Here's how the part is built. I have some questions about the finished solid (model axes, mm). A direction names the side the tool comes from. Coordinates: 2 decimals unless noted, no trailing zeros. Order: outer loops, then holes, each group sorted by start corner. A loop starts at its lowest first (then second) coordinate and runs counter-clockwise, first axis right, second up. Notation, with made-up numbers: (-37.5, 69) - (-8.5, 69) arc R26 cw to (-8.5, 88) - close; hole circle Ø1 at (69.25, 15.5). An arc over 180 degrees is marked (long way). Answer as CSV lines item,"result". Start each with the question number.
Q1. For faces 1 (the face through (1, 46, 35)), 2 (the face through (-31.27, 39.03, 36.59)), which set-ups out of +Z, -Z, +X, -X, +Y, -Y let a thin tool reach every point of the face, with its end or its side?
Q2. For pin 1 Ø3.5 at (x, y) = (-45.75, 40) entering from +Z; pin 2 Ø10 at (x, y) = (-15, -26.5) entering from -Z, each with a flat end and sliding along its axis, tell me the tip position at first contact or that it passes through.
Q3. Suppose I cut it at B-B (x = 45.75). Please give me the cut outline in (y, z), then the cut area to 3 significant figures.
Q4. Suppose I cut it at C-C (z = 34.4). Please give me the cut outline in (x, y).
Q5. Suppose I cut it at D-D (y = 40). Please give me the cut outline in (x, z), then the cut area to 3 significant figures.
Q6. I need wall thicknesses on line 1 (X direction, y = -42, z = 36.5); line 2 (Y direction, x = -30, z = 36.6); line 3 (Y direction, x = 33, z = 33.95). Which ranges of each line are inside material? Lowest first, please.
Q7. Suppose I cut it at A-A (y = -42). Please give me the cut outline in (x, z).
Q8. Thinking about a two-plate mould opening in Y: for faces 3 (the face through (-1, -47, 35)), 4 (the face through (1, 47, 35)), 5 (the face through (-50.75, 1, 35)), 6 (the face through (49.75, -1, 35)), which applies, released by +Y, released by -Y, zero draft, split by the parting line, or undercut?
from build123d import *

# Parameters (mm, degrees)
PAD024_DEPTH    = 1
PAD025_DEPTH    = 3
SKETCH042_R     = 1.6
POCKET018_DEPTH = 5


with BuildPart() as part:
    # Sketch040 → Pad024 (new body)
    with BuildSketch(Plane.XY):
        with BuildLine():
            Line((-50.75, 46), (-50.75, -46))
            ThreePointArc((-50.75, -46), (-50.457107, -46.707107), (-49.75, -47))
            Line((-49.75, -47), (49.75, -47))
            ThreePointArc((49.75, -47), (50.457107, -46.707107), (50.75, -46))
            Line((50.75, -46), (50.75, 46))
            ThreePointArc((50.75, 46), (50.457107, 46.707107), (49.75, 47))
            Line((49.75, 47), (-49.75, 47))
            ThreePointArc((-49.75, 47), (-50.457107, 46.707107), (-50.75, 46))
        make_face()
    extrude(amount=PAD024_DEPTH)

    # Sketch041 → Pad025 (join)
    with BuildSketch(Plane.XY):
        with BuildLine():
            Line((-50.75, 46), (-50.75, -46))
            ThreePointArc((-50.75, -46), (-50.457107, -46.707107), (-49.75, -47))
            Line((-49.75, -47), (49.75, -47))
            ThreePointArc((49.75, -47), (50.457107, -46.707107), (50.75, -46))
            Line((50.75, -46), (50.75, 46))
            ThreePointArc((50.75, 46), (50.457107, 46.707107), (49.75, 47))
            Line((49.75, 47), (-49.75, 47))
            ThreePointArc((-49.75, 47), (-50.457107, 46.707107), (-50.75, 46))
        make_face()
        with BuildLine():
            Line((-49.75, 45), (-49.75, -45))
            ThreePointArc((-49.75, -45), (-49.457107, -45.707107), (-48.75, -46))
            Line((-48.75, -46), (48.75, -46))
            ThreePointArc((48.75, -46), (49.457107, -45.707107), (49.75, -45))
            Line((49.75, -45), (49.75, 45))
            ThreePointArc((49.75, 45), (49.457107, 45.707107), (48.75, 46))
            Line((48.75, 46), (-48.75, 46))
            ThreePointArc((-48.75, 46), (-49.457107, 45.707107), (-49.75, 45))
        make_face(mode=Mode.SUBTRACT)
    extrude(amount=-PAD025_DEPTH)

    # Sketch042 → Pocket018 (cut)
    with BuildSketch(Plane.XY):
        with Locations((-45.75, 40)):
            Circle(SKETCH042_R)
        with Locations((-30, 40)):
            Circle(SKETCH042_R)
        with Locations((30, 40)):
            Circle(SKETCH042_R)
        with Locations((-30, -42)):
            Circle(SKETCH042_R)
        with Locations((-45.75, -42)):
            Circle(SKETCH042_R)
        with Locations((30, -42)):
            Circle(SKETCH042_R)
        with Locations((45.75, -42)):
            Circle(SKETCH042_R)
    extrude(amount=POCKET018_DEPTH, mode=Mode.SUBTRACT)


with BuildPart() as part_1:
    # Body010 placement: moved
    add(part.part.moved(Location((0, 0, 36.1))))


solid = part_1.part
Here are the results:
1,face 1,"-Z"
1,face 2,"+Z, -Z"
2,pin 1,"stops at z = 37.1"
2,pin 2,"stops at z = 36.1"
3,outline,"(-47, 33.1) - (-46, 33.1) - (-46, 36.1) - (-43.6, 36.1) - (-43.6, 37.1) - (-47, 37.1) - close; (-40.4, 36.1) - (46, 36.1) - (46, 33.1) - (47, 33.1) - (47, 37.1) - (-40.4, 37.1) - close"
3,area,"96.8 mm²"
4,outline,"(-50.75, -46) arc R1 ccw to (-49.75, -47) - (49.75, -47) arc R1 ccw to (50.75, -46) - (50.75, 46) arc R1 ccw to (49.75, 47) - (-49.75, 47) arc R1 ccw to (-50.75, 46) - close; hole (-49.75, -45) arc R1 ccw to (-48.75, -46) - (48.75, -46) arc R1 ccw to (49.75, -45) - (49.75, 45) arc R1 ccw to (48.75, 46) - (-48.75, 46) arc R1 ccw to (-49.75, 45) - close"
5,outline,"(-50.75, 33.1) - (-49.75, 33.1) - (-49.75, 36.1) - (-47.35, 36.1) - (-47.35, 37.1) - (-50.75, 37.1) - close; (-44.15, 36.1) - (-31.6, 36.1) - (-31.6, 37.1) - (-44.15, 37.1) - close; (-28.4, 36.1) - (28.4, 36.1) - (28.4, 37.1) - (-28.4, 37.1) - close; (31.6, 36.1) - (49.75, 36.1) - (49.75, 33.1) - (50.75, 33.1) - (50.75, 37.1) - (31.6, 37.1) - close"
5,area,"97.9 mm²"
6,line 1,"x = -50.75 to -47.35, -44.15 to -31.6, -28.4 to 28.4, 31.6 to 44.15, 47.35 to 50.75"
6,line 2,"y = -47 to -43.6, -40.4 to 38.4, 41.6 to 47"
6,line 3,"y = -47 to -46, 46 to 47"
7,outline,"(-50.75, 33.1) - (-49.75, 33.1) - (-49.75, 36.1) - (-47.35, 36.1) - (-47.35, 37.1) - (-50.75, 37.1) - close; (-44.15, 36.1) - (-31.6, 36.1) - (-31.6, 37.1) - (-44.15, 37.1) - close; (-28.4, 36.1) - (28.4, 36.1) - (28.4, 37.1) - (-28.4, 37.1) - close; (31.6, 36.1) - (44.15, 36.1) - (44.15, 37.1) - (31.6, 37.1) - close; (47.35, 36.1) - (49.75, 36.1) - (49.75, 33.1) - (50.75, 33.1) - (50.75, 37.1) - (47.35, 37.1) - close"
8,face 3,"released by -Y"
8,face 4,"released by +Y"
8,face 5,"zero draft"
8,face 6,"undercut"
